Geometry check sheet. Reference: the model listing, model coordinates, mm. Face numbers are marked on the shaded views. A direction names the side the tool comes from. Coordinates: 2 decimals unless noted, no trailing zeros. Loops run counter-clockwise (first coordinate to the right, second up) from the corner with the lowest first, then second, coordinate; pieces in that order, holes last. Notation, with made-up numbers: (34, 60.25) -> (60, 60.25) arc R35 cw to (60, 93.25) -> close; hole circle Ø11 at (-28, 73.5). An arc over 180 degrees is marked (long way). Answer as a JSON object with one key per item and string values.
from build123d import *

# Parameters (mm, degrees)
BOSS_EXTRUDE1_DEPTH = 11.43
SKETCH3_R           = 2.75
CUT_EXTRUDE1_DEPTH  = 71.56504464
SKETCH4_R           = 2.75
CUT_EXTRUDE2_DEPTH  = 71.56504464


with BuildPart() as part:
    # Sketch2 → Boss-Extrude1 (new, symmetric)
    with BuildSketch(Plane.XY):
        with BuildLine():
            Line((0, 0), (0, -50.8))
            Line((0, -50.8), (50.8, -50.8))
            Line((50.8, -50.8), (50.8, -47.625))
            Line((50.8, -47.625), (5.715, -47.625))
            ThreePointArc((5.715, -47.625), (3.918948776, -46.881051224), (3.175, -45.085))
            Line((3.175, -45.085), (3.175, 0))
            Line((3.175, 0), (0, 0))
        make_face()
    extrude(amount=BOSS_EXTRUDE1_DEPTH, both=True)

    # Sketch3 → Cut-Extrude1 (cut, through all)
    with BuildSketch(Plane(origin=(3.175, 0, 0), x_dir=(0, 0, -1), z_dir=(1, 0, 0))):
        with Locations(Location((0, -5.08, 0), (0, 0, 90))):
            Circle(SKETCH3_R)
        with Locations(Location((0, -17.78, 0), (0, 0, 90))):
            Circle(SKETCH3_R)
    extrude(amount=-CUT_EXTRUDE1_DEPTH, mode=Mode.SUBTRACT)

    # Sketch4 → Cut-Extrude2 (cut, through all)
    with BuildSketch(Plane(origin=(0, -47.625, 0), x_dir=(1, 0, 0), z_dir=(0, 1, 0))):
        with Locations(Location((19.812, 0, 0), (0, 0, 270))):
            Circle(SKETCH4_R)
        with Locations(Location((45.72, 0, 0), (0, 0, 270))):
            Circle(SKETCH4_R)
    extrude(amount=-CUT_EXTRUDE2_DEPTH, mode=Mode.SUBTRACT)


solid = part.part
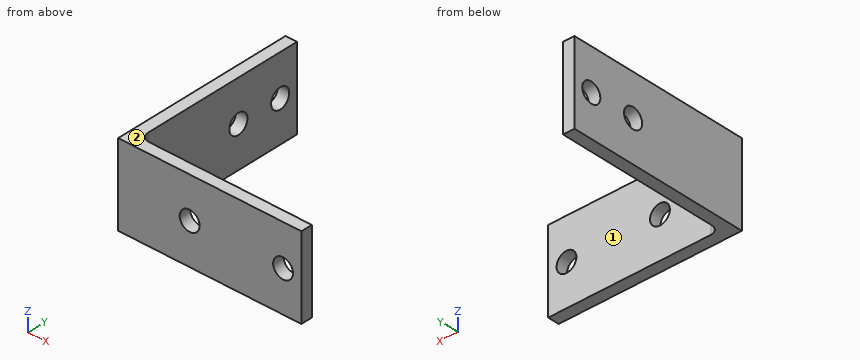
1. Thickness scan on probe 1 along X at (y, z) = (-28, -2.25) (3 decimals); probe 2 along Y at (x, z) = (5.5, 3); probe 3 along Z at (x, y) = (3, -18.5). Record the ranges inside material, lowest first. Write a range as from..to.
Evaluation:
{"probe 1": "x = 0..3.175", "probe 2": "y = -50.8..-47.62", "probe 3": "z = -11.43..-2.65, 2.65..11.43"}
2. Section check A-A, the plane x = 45.72. Record the boundary of the cut face in (y, z) (3 decimals).
Evaluation:
{"outline": "(-50.8, -11.43) -> (-47.625, -11.43) -> (-47.625, -2.75) -> (-50.8, -2.75) -> close; (-50.8, 2.75) -> (-47.625, 2.75) -> (-47.625, 11.43) -> (-50.8, 11.43) -> close"}
3. Tool access check on the marked faces 1 and 2. Record the directions out of +Z, -Z, +X, -X, +Y, -Y that give a thin tool (end or side, any length) a straight path to the whole face; none if there is none.
Evaluation:
{"face 1": "+Z, -Z, +X, +Y", "face 2": "+Z, +X, -X, +Y, -Y"}
4. Section check B-B, the plane z = 0. Record the boundary of the cut face in (x, y) (3 decimals).
Evaluation:
{"outline": "(0, -50.8) -> (17.062, -50.8) -> (17.062, -47.625) -> (5.715, -47.625) arc R2.54 cw to (3.175, -45.085) -> (3.175, -20.53) -> (0, -20.53) -> close; (0, -15.03) -> (3.175, -15.03) -> (3.175, -7.83) -> (0, -7.83) -> close; (0, -2.33) -> (3.175, -2.33) -> (3.175, 0) -> (0, 0) -> close; (22.562, -50.8) -> (42.97, -50.8) -> (42.97, -47.625) -> (22.562, -47.625) -> close; (48.47, -50.8) -> (50.8, -50.8) -> (50.8, -47.625) -> (48.47, -47.625) -> close"}
5. Depth check by flat-ended pin: P1, Ø6, axis at y = -25.5, z = -7.5, coming from the +X side (3 decimals); P2, Ø10, axis at x = 14.5, z = -5, coming from the +Y side (3 decimals); P3, Ø3.5, axis at x = 45.72, z = 0, coming from the -Y side. Enter the tip coordinate at first touch or a pass-through.
Evaluation:
{"P1": "stops at x = 3.175", "P2": "stops at y = -47.625", "P3": "passes through"}
6. Section check D-D, the plane z = -4.75. Record the boundary of the cut face in (x, y) (3 decimals).
Evaluation:
{"outline": "(0, -50.8) -> (50.8, -50.8) -> (50.8, -47.625) -> (5.715, -47.625) arc R2.54 cw to (3.175, -45.085) -> (3.175, 0) -> (0, 0) -> close"}
7. Section check C-C, the plane y = -17.78. Record the boundary of the cut face in (x, z) (3 decimals).
Evaluation:
{"outline": "(0, -11.43) -> (3.175, -11.43) -> (3.175, -2.75) -> (0, -2.75) -> close; (0, 2.75) -> (3.175, 2.75) -> (3.175, 11.43) -> (0, 11.43) -> close"}
